Check sheet for the modelled part. Datum: model origin and axes. Units: mm. A direction names the side the tool comes from. Give positions to 0.01 mm unless a question says otherwise; leave off trailing zeros. Order: outer loops, then holes, each group sorted by start corner. A loop starts at its lowest first (then second) coordinate and runs counter-clockwise, first axis right, second up. Notation, with made-up numbers: (-39.75, -33) - (5.25, -33) arc R24 ccw to (5.25, -12) - close; hole circle Ø6 at (-21, 48). An arc over 180 degrees is marked (long way). Answer in a Markdown table with one row per item.
from build123d import *

# Parameters (mm, degrees)
BOSS_EXTRUDE1_DEPTH = 2.5
SKETCH2_R           = 1.78
CUT_EXTRUDE1_DEPTH  = 1.5
FILLET1_R           = 1.5


with BuildPart() as part:
    # Sketch1 → Boss-Extrude1 (new body)
    with BuildSketch(Plane(origin=(0, 0, 0), x_dir=(1, 0, 0), z_dir=(0, 1, 0))):
        Polygon((-21.216153836, 11.741903429), (-21.216153836, 8.241903429), (-8.076153836, -0.958096571), (-2.716153836, -0.958096571), (-2.716153836, 11.741903429), align=None)
    extrude(amount=BOSS_EXTRUDE1_DEPTH)

    # Sketch2 → Cut-Extrude1 (cut)
    with BuildSketch(Plane(origin=(0, 2.5, 0), x_dir=(1, 0, 0), z_dir=(0, 1, 0))):
        with Locations((-17.966153836, 8.241903429)):
            Circle(SKETCH2_R)
    extrude(amount=-CUT_EXTRUDE1_DEPTH, mode=Mode.SUBTRACT)

    # Fillet1
    fillet1_edges = [part.edges().sort_by_distance(p)[0] for p in [
        (-5.396153836, 0, 0.958096571),
        (-14.646153836, 0, -3.641903429),
        (-21.216153836, 0, -9.991903429),
        (-11.966153836, 0, -11.741903429),
        (-8.076153836, 1.25, 0.958096571),
        (-21.216153836, 1.25, -8.241903429),
        (-21.216153836, 1.25, -11.741903429),
    ]]
    fillet(fillet1_edges, radius=FILLET1_R)

    # Mirror1: part across plane


with BuildPart() as part_1:
    add(part.part)
    add(part.part.mirror(Plane(origin=(-2.716153836, 2.5, 0.958096571), x_dir=(0, 0, 1), z_dir=(-1, 0, 0))))


solid = part_1.part
(1) Access from +Z, -Z, +X, -X, +Y, -Y to the whole of each face (thin tool, end or side, straight path). Record for faces 1 (the flat face through (15.784, 2, -10)), 2 (the cylindrical face through (10.836, 1.76, -8.777)).
Geometry says:
| item | result |
|---|---|
| face 1 | +Z, -Z, +X, +Y, -Y |
| face 2 | +Y |
(2) Gauge pin test, flat ends, axial feed: P1, Ø1.8, axis at x = -18.5, z = -7.5, coming from the +Y side; P2, Ø1.5, axis at x = 10.5, y = 2, coming from the +Z side; P3, Ø6, axis at x = -14, z = -0.5, coming from the -Y side (3 decimals). Record the tip position at first contact, or that the pin passes through.
Geometry says:
| item | result |
|---|---|
| P1 | y = 2.5 |
| P2 | z = -4.02 |
| P3 | y = 0.175 |
(3) Cross-section at B-B, the plane x = -3. Record the cut outline in (y, z).
Geometry says:
| item | result |
|---|---|
| outline | (0, -10.24) arc R1.5 ccw to (1.5, -11.74) - (2.5, -11.74) - (2.5, 0.96) - (1.5, 0.96) arc R1.5 ccw to (0, -0.54) - close |
(4) Mould release check, pull along Z, two halves, no side actions. Record for faces 3 (the cylindrical face through (15.356, 2.007, -11.291)), 4 (the flat face through (-21.216, 2, -10)), 5 (the cylindrical face through (-17.009, 1.76, -9.743)), 6 (the flat face through (-18, 1, -8)): pulls with the +Z half, pulls with the -Z half, needs draft (parallel to the pull), parting line crosses it, or undercut.
Geometry says:
| item | result |
|---|---|
| face 3 | pulls with the -Z half |
| face 4 | needs draft |
| face 5 | undercut |
| face 6 | undercut |
(5) Thickness scan on L1, parallel to Z at x = 11, y = 1.25; L2, parallel to Z at x = 12.5, y = 1.45; L3, parallel to X at y = 2.05, z = -1.75. Record the ranges inside material, lowest first.
Geometry says:
| item | result |
|---|---|
| L1 | -11.72 to -9.15, -7.34 to -4.92 |
| L2 | -11.74 to -10.02, -6.46 to -5.94 |
| L3 | -11.94 to 6.51 |
(6) Cross-section at A-A, the plane y = 0.45. Record the cut outline in (x, z), then the cut area to 3 significant figures.
Geometry says:
| item | result |
|---|---|
| outline | (-20.79, -10.24) arc R1.07 ccw to (-19.72, -11.31) - (14.28, -11.31) arc R1.07 ccw to (15.36, -10.24) - (15.36, -9.02) arc R1.07 ccw to (14.9, -8.15) - (2.79, 0.34) arc R1.07 ccw to (2.17, 0.53) - (-7.6, 0.53) arc R1.07 ccw to (-8.22, 0.34) - (-20.33, -8.15) arc R1.07 ccw to (-20.79, -9.02) - close |
| area | 312 mm² |
